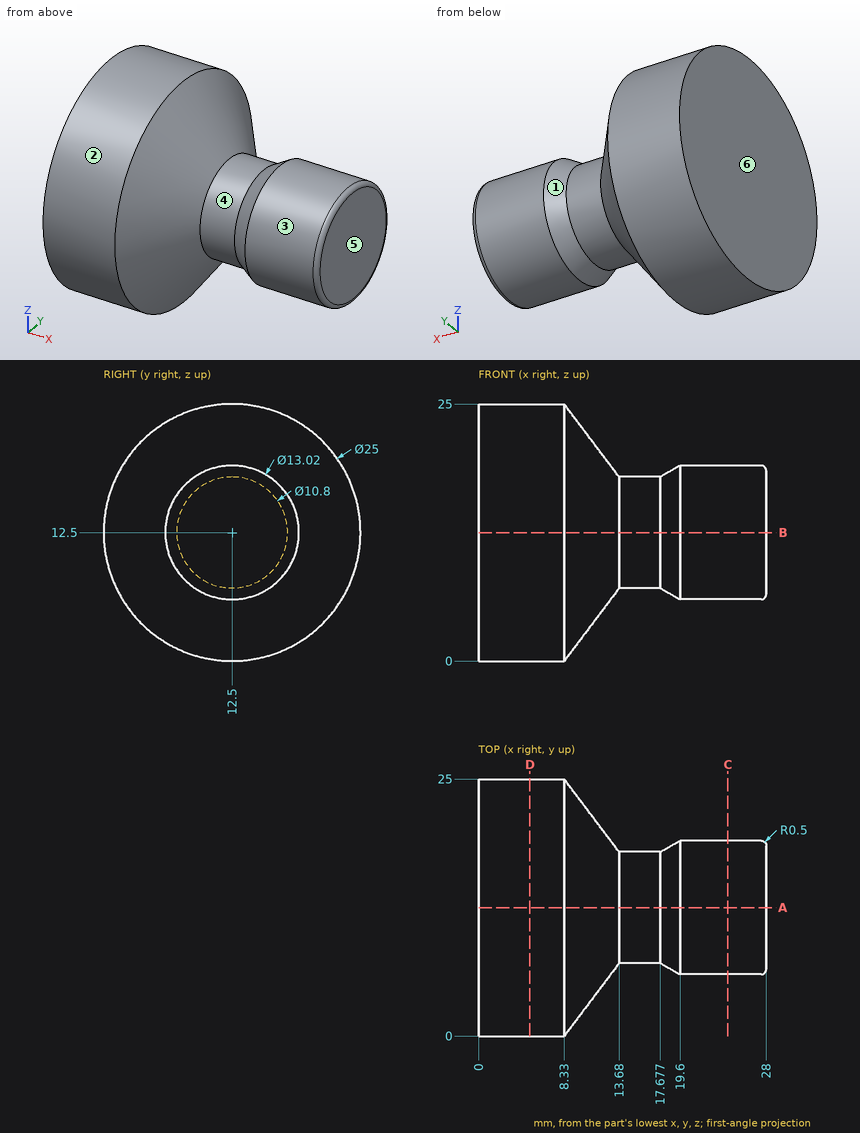
Could you check a few things on this drawing? It's one solid part, dimensions in mm from its lowest x, y, z. A direction names the side the tool comes from. Give positions to 0.01 mm unless a question says otherwise; leave off trailing zeros. Write each loop counter-clockwise with the first axis right and the second up, starting at its lowest first coordinate (ties: lowest second). Pieces come first, ordered by that corner, then holes. Notation, with made-up numbers: M -16,19 L 27,19 A19 cw 27,27 Z; hole C -27.5,41 d5. An arc over 180 degrees is marked long. Put each result on its own line as item: value. Start each with the question number.
Item 1: On a 3-axis mill with a long thin cutter (end or side, diameter ignored), from which of +Z, -Z, +X, -X, +Y, -Y can I reach the whole of each face in a straight line? I mean the marked faces 1, 2 and 3. Say none if no direction works.
Item 2: Will these pins go through, and if not, where does the flat tip stop? pin 1 (3 mm diameter, centred on x = 3.5, y = 19, fed in from -Z); pin 2 (12 mm diameter, centred on x = 22, z = 18, fed in from -Y); pin 3 (1.5 mm diameter, centred on x = 25, z = 10, fed in from -Y).
Item 3: If we section it at C-C, the plane x = 24.25: Write out the boundary of the cut face in (y, z).
Item 4: Thinking about a two-plate mould opening in X: for the marked faces 4, 5 and 6, which applies, +X half, -X half, draft (parallel to the pull), parting line (faces both ways), or undercut?
Item 5: If we section it at D-D, the plane x = 5: Write out the boundary of the cut face in (y, z), then the cut area to 3 significant figures.
Item 6: If we section it at A-A, the plane y = 12.5: Write out the boundary of the cut face in (x, z).
Item 7: I need wall thicknesses on L1, parallel to X at y = 16.5, z = 17.25; L2, parallel to Y at x = 8, z = 17.25; L3, parallel to Y at x = 23.25, z = 11.25. Which ranges of each line are inside material? Lowest first, please. Write a range as from..to.
Values:
1. face 1: none
1. face 2: +X, -X
1. face 3: +X
2. pin 1: z = 1.04
2. pin 2: y = 5.99
2. pin 3: y = 6.23
3. outline: C 12.5,12.5 d13.02
4. face 4: undercut
4. face 5: +X half
4. face 6: -X half
5. outline: C 12.5,12.5 d25
5. area: 491 mm²
6. outline: M 0,0 L 8.33,0 L 13.68,7.1 L 17.68,7.1 L 19.6,5.99 L 27.5,5.99 A0.5 ccw 28,6.49 L 28,18.51 A0.5 ccw 27.5,19.01 L 19.6,19.01 L 17.68,17.9 L 13.68,17.9 L 8.33,25 L 0,25 Z
7. L1: 0..13.07, 19.08..27.96
7. L2: 0.94..24.06
7. L3: 6.11..18.89
